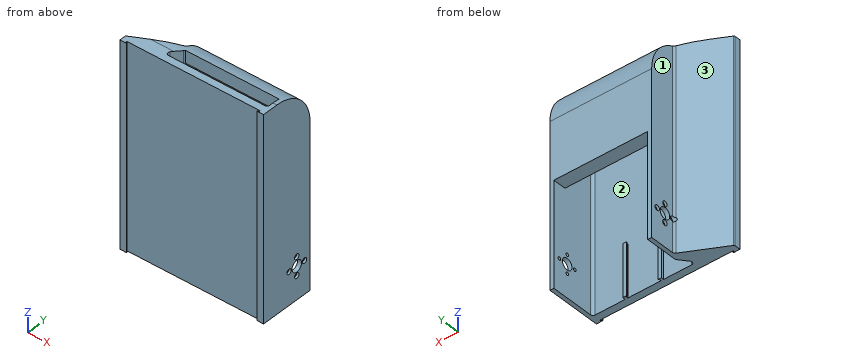
from build123d import *

# Parameters (mm, degrees)
BOSS_EXTRUDE1_DEPTH = 155
SKETCH3_R           = 4.3
SKETCH3_R_2         = 1.2
CUT_EXTRUDE1_DEPTH  = 3
SKETCH2_R           = 4.3
SKETCH2_R_2         = 1.1
CUT_EXTRUDE2_DEPTH  = 178.191866295
SKETCH4_R           = 2
CUT_EXTRUDE3_DEPTH  = 1.7
CUT_EXTRUDE4_START  = -1.7
SKETCH5_R           = 2
CUT_EXTRUDE4_DEPTH  = 1.7
CUT_EXTRUDE5_START  = -1.7
SKETCH5_4_R         = 2
CUT_EXTRUDE5_DEPTH  = 181.180461853
FILLET1_R           = 2
FILLET2_R           = 1
BOSS_EXTRUDE3_DEPTH = 71.886297018
FILLET3_R           = 30
BOSS_EXTRUDE4_DEPTH = 40


with BuildPart() as part:
    # Sketch1 → Boss-Extrude1 (new body)
    with BuildSketch(Plane.XY):
        Polygon((29.816959294, 42), (29.816959294, 17), (21.703256312, 7), (101.703256312, 7), (101.703256312, 42), (104.703256312, 42), (104.703256312, 14.387755102), (104.703256312, 0), (99.703256312, 0), (99.703256312, 0.5), (100.703256312, 0.5), (100.703256312, 1.5), (-1.296743688, 1.5), (-1.296743688, 0.5), (-0.296743688, 0.5), (-0.296743688, 0), (-5.296743688, 0), (-5.296743688, 5), (26.816959294, 22), (26.816959294, 42), align=None)
    extrude(amount=BOSS_EXTRUDE1_DEPTH)

    # Sketch3 → Cut-Extrude1 (cut)
    with BuildSketch(Plane.ZY.offset(-101.703256312)):
        with Locations((25, 30)):
            Circle(SKETCH3_R)
        with Locations((25, 37)):
            Circle(SKETCH3_R_2)
        with Locations((32, 30)):
            Circle(SKETCH3_R_2)
        with Locations((25, 23)):
            Circle(SKETCH3_R_2)
        with Locations((18, 30)):
            Circle(SKETCH3_R_2)
    extrude(amount=-CUT_EXTRUDE1_DEPTH, mode=Mode.SUBTRACT)

    # Sketch2 → Cut-Extrude2 (cut, through all)
    with BuildSketch(Plane(origin=(29.816959294, 0, 0), x_dir=(0, 0, -1), z_dir=(1, 0, 0))):
        with Locations(Location((-25, 30, 0), (0, 0, 180))):
            Circle(SKETCH2_R)
        with Locations(Location((-25, 37, 0), (0, 0, 90))):
            Circle(SKETCH2_R_2)
        with Locations(Location((-18, 30, 0), (0, 0, 90))):
            Circle(SKETCH2_R_2)
        with Locations(Location((-25, 23, 0), (0, 0, 90))):
            Circle(SKETCH2_R_2)
        with Locations(Location((-32, 30, 0), (0, 0, 90))):
            Circle(SKETCH2_R_2)
    extrude(amount=-CUT_EXTRUDE2_DEPTH, mode=Mode.SUBTRACT)

    # Sketch4 → Cut-Extrude3 (cut)
    with BuildSketch(Plane(origin=(104.703256312, 0, 0), x_dir=(0, 0, -1), z_dir=(1, 0, 0))):
        with Locations(Location((-32, 30, 0), (0, 0, 90))):
            Circle(SKETCH4_R)
        with Locations(Location((-25, 37, 0), (0, 0, 90))):
            Circle(SKETCH4_R)
        with Locations(Location((-18, 30, 0), (0, 0, 90))):
            Circle(SKETCH4_R)
        with Locations(Location((-25, 23, 0), (0, 0, 90))):
            Circle(SKETCH4_R)
    extrude(amount=-CUT_EXTRUDE3_DEPTH, mode=Mode.SUBTRACT)

    # Sketch5 → Cut-Extrude4 (cut)
    with BuildSketch(Plane.ZY.offset(-26.816959294).offset(CUT_EXTRUDE4_START)):
        with Locations(Location((25, 23, 0), (0, 0, 90))):
            Circle(SKETCH5_R)
        with Locations(Location((32, 30, 0), (0, 0, 90))):
            Circle(SKETCH5_R)
        with Locations(Location((25, 37, 0), (0, 0, 90))):
            Circle(SKETCH5_R)
        with Locations(Location((18, 30, 0), (0, 0, 90))):
            Circle(SKETCH5_R)
    extrude(amount=CUT_EXTRUDE4_DEPTH, mode=Mode.SUBTRACT)

    # Sketch5<4> → Cut-Extrude5 (cut, through all)
    with BuildSketch(Plane.ZY.offset(-26.816959294).offset(CUT_EXTRUDE5_START)):
        with Locations(Location((25, 23, 0), (0, 0, 90))):
            Circle(SKETCH5_4_R)
        with Locations(Location((32, 30, 0), (0, 0, 90))):
            Circle(SKETCH5_4_R)
        with Locations(Location((25, 37, 0), (0, 0, 90))):
            Circle(SKETCH5_4_R)
        with Locations(Location((18, 30, 0), (0, 0, 90))):
            Circle(SKETCH5_4_R)
    extrude(amount=CUT_EXTRUDE5_DEPTH, mode=Mode.SUBTRACT)

    # Fillet1
    fillet1_edges = [part.edges().sort_by_distance(p)[0] for p in [
        (101.703256312, 7, 77.5),
        (29.816959294, 17, 77.5),
        (21.703256312, 7, 77.5),
        (26.816959294, 22, 11.633974596),
        (26.816959294, 22, 90.866025404),
    ]]
    fillet(fillet1_edges, radius=FILLET1_R)

    # Fillet2
    fillet2_edges = [part.edges().sort_by_distance(p)[0] for p in [
        (-5.296743688, 5, 77.5),
    ]]
    fillet(fillet2_edges, radius=FILLET2_R)

    # Sketch8 → Boss-Extrude3 (add)
    with BuildSketch(Plane(origin=(29.816959294, 0, 0), x_dir=(0, 0, -1), z_dir=(1, 0, 0))):
        with BuildLine():
            Line((-155, 42), (-155, 17.709314663))
            Line((-155, 17.709314663), (-145, 17.709314663))
            ThreePointArc((-145, 17.709314663), (-114.980171869, 36.135513896), (-80, 32))
            Line((-80, 32), (-80, 42))
            Line((-80, 42), (-155, 42))
        make_face()
    extrude(amount=BOSS_EXTRUDE3_DEPTH)

    # Fillet3
    # the kernel refuses this fillet: 30 mm, written as the material it takes off along each edge
    with BuildSketch(Plane(origin=(-48.183040706, 42, 155), x_dir=(0, -1, 0), z_dir=(1, 0, 0))) as fillet3_piece_1:
        with BuildLine():
            CenterArc((FILLET3_R, FILLET3_R), FILLET3_R, 180, 90)
            Line((0, FILLET3_R), (0, 0))
            Line((0, 0), (FILLET3_R, 0))
        make_face()
    extrude(amount=227.886297018, mode=Mode.SUBTRACT)

    # Sketch10 → Boss-Extrude4 (add)
    with BuildSketch(Plane(origin=(0, 0, 0), x_dir=(-1, 0, 0), z_dir=(0, 0, -1))):
        Polygon((-74.703256312, 7), (-74.703256312, 8.6), (-74.103256312, 8.6), (-74.103256312, 9.1), (-76.703256312, 9.1), (-76.703256312, 7), align=None)
        Polygon((-47.303256312, 7), (-47.303256312, 9.1), (-49.903256312, 9.1), (-49.903256312, 8.6), (-49.303256312, 8.6), (-49.303256312, 7), align=None)
    extrude(amount=-BOSS_EXTRUDE4_DEPTH)


solid = part.part
Model file for the job. Use its own axes, mm. Face numbers are marked on the shaded views. Round coordinates to 2 decimals unless told otherwise and drop trailing zeros. Loops run counter-clockwise (first coordinate to the right, second up) from the corner with the lowest first, then second, coordinate; pieces in that order, holes last. Notation, with made-up numbers: (21.25, 12) -> (52.25, 12) arc R16 ccw to (52.25, 31) -> close; hole circle Ø3 at (13.5, -27). An arc over 180 degrees is marked (long way). Answer as CSV lines item,"result". Start each with the question number.
1) Probe line 1 along X through (y, z) = (32, 121.5); line 2 along Y through (x, z) = (28, 18); line 3 along X through (y, z) = (20, 83). List the from-to ranges inside material, lowest first.
2) Slice it at A-A (z = 71). List the corners of the cut face in (x, y).
3) Slice it at C-C (z = 98). List the corners of the cut face in (x, y), plus the area to 3 significant figures.
4) Pin check, flat tips, straight feed: P1, Ø3, axis at y = 34.5, z = 21.5, coming from the -X side; P2, Ø0.6, axis at x = 49, y = 8, coming from the +Z side; P3, Ø3, axis at x = 22, z = 82.5, coming from the +Y side. Stop position of each tip, or through.
5) Mould opens along Y. For the marked faces 1, 2 and 3 say: +Y half, -Y half, draft (parallel to the pull), parting line (faces both ways), or undercut.
6) Slice it at D-D (x = 12.5). List the corners of the cut face in (y, z), plus the area to 3 significant figures.
7) Slice it at B-B (x = 83). List the corners of the cut face in (y, z), plus the area to 3 significant figures.
Filled in:
1,line 1,"x = 26.82 to 29.82, 101.7 to 104.7"
1,line 2,"y = 1.5 to 7, 14.76 to 28, 32 to 42"
1,line 3,"x = 23.04 to 29.82, 101.7 to 104.7"
2,outline,"(-5.3, 0) -> (-0.3, 0) -> (-0.3, 0.5) -> (-1.3, 0.5) -> (-1.3, 1.5) -> (100.7, 1.5) -> (100.7, 0.5) -> (99.7, 0.5) -> (99.7, 0) -> (104.7, 0) -> (104.7, 42) -> (101.7, 42) -> (101.7, 9) arc R2 cw to (99.7, 7) -> (25.9, 7) arc R2 cw to (24.35, 10.26) -> (29.37, 16.45) arc R2 ccw to (29.82, 17.71) -> (29.82, 42) -> (26.82, 42) -> (26.82, 23.2) arc R2 cw to (25.75, 21.44) -> (-4.76, 5.28) arc R1 ccw to (-5.3, 4.4) -> close"
3,outline,"(-5.3, 0) -> (-0.3, 0) -> (-0.3, 0.5) -> (-1.3, 0.5) -> (-1.3, 1.5) -> (100.7, 1.5) -> (100.7, 0.5) -> (99.7, 0.5) -> (99.7, 0) -> (104.7, 0) -> (104.7, 42) -> (26.82, 42) -> (26.82, 23.2) arc R2 cw to (25.75, 21.44) -> (-4.76, 5.28) arc R1 ccw to (-5.3, 4.4) -> close; hole (24.35, 10.26) arc R2 ccw to (25.9, 7) -> (99.7, 7) arc R2 ccw to (101.7, 9) -> (101.7, 37.11) -> (29.82, 37.11) -> (29.82, 17.71) arc R2 cw to (29.37, 16.45) -> close"
3,area,"1,350 mm2"
4,P1,"stops at x = 26.82"
4,P2,"stops at z = 40"
4,P3,"stops at y = 20.24"
5,face 1,"draft"
5,face 2,"undercut"
5,face 3,"+Y half"
6,outline,"(1.5, 0) -> (14.42, 0) -> (14.42, 154.9) arc R30 ccw to (12, 155) -> (1.5, 155) -> close"
6,area,"2,000 mm2"
7,outline,"(1.5, 0) -> (7, 0) -> (7, 155) -> (1.5, 155) -> close; (17.71, 145) arc R53.71 cw to (32, 80) -> (42, 80) -> (42, 125) arc R30 ccw to (17.71, 154.45) -> close"
7,area,"1,490 mm2"
